from build123d import *

# Parameters (mm, degrees)
BOSS_EXTRUDE2_DEPTH = 48.5
BOSS_EXTRUDE3_DEPTH = 18
SKETCH3_R           = 1.6
CUT_EXTRUDE1_DEPTH  = 8
CUT_EXTRUDE3_DEPTH  = 3
SKETCH5_W           = 78.5
SKETCH5_H           = 16
BOSS_EXTRUDE4_DEPTH = 2
BOSS_EXTRUDE5_DEPTH = 7
BOSS_EXTRUDE6_DEPTH = 7
SKETCH10_R          = 2.1
CUT_EXTRUDE4_DEPTH  = 17
CUT_EXTRUDE5_DEPTH  = 3
CUT_EXTRUDE6_DEPTH  = 8


with BuildPart() as part:
    # Sketch1 → Boss-Extrude2 (new body)
    with BuildSketch(Plane.XY):
        with BuildLine():
            ThreePointArc((-2.027849528, -2.111075236), (-1.295616481, -3.878842189), (0.472150472, -4.611075236))
            Line((0.472150472, -4.611075236), (0.472150472, -7.611075236))
            Line((0.472150472, -7.611075236), (-17.527849528, -7.611075236))
            Line((-17.527849528, -7.611075236), (-17.527849528, 8.388924764))
            Line((-17.527849528, 8.388924764), (0.472150472, 8.388924764))
            Line((0.472150472, 8.388924764), (0.472150472, 5.388924764))
            ThreePointArc((0.472150472, 5.388924764), (-1.295616481, 4.656691717), (-2.027849528, 2.888924764))
            Line((-2.027849528, 2.888924764), (-2.027849528, -2.111075236))
        make_face()
    extrude(amount=BOSS_EXTRUDE2_DEPTH)

    # Sketch2 → Boss-Extrude3 (add)
    with BuildSketch(Plane.ZY.offset(17.527849528)):
        with BuildLine():
            Line((48.5, 8.388924764), (62.5, 8.388924764))
            Line((62.5, 8.388924764), (63.5, 8.388924764))
            Line((63.5, 8.388924764), (63.5, 7.388924764))
            Line((63.5, 7.388924764), (63.5, -6.611075236))
            Line((63.5, -6.611075236), (63.5, -7.611075236))
            Line((63.5, -7.611075236), (62.5, -7.611075236))
            Line((62.5, -7.611075236), (48.5, -7.611075236))
            Line((48.5, -7.611075236), (48.5, -4.811075236))
            Line((48.5, -4.811075236), (58.6, -4.811075236))
            ThreePointArc((58.6, -4.811075236), (58.670710678, -4.781785914), (58.7, -4.711075236))
            Line((58.7, -4.711075236), (58.7, 5.488924764))
            ThreePointArc((58.7, 5.488924764), (58.670710678, 5.559635442), (58.6, 5.588924764))
            Line((58.6, 5.588924764), (48.5, 5.588924764))
            Line((48.5, 5.588924764), (48.5, 8.388924764))
        make_face()
        with BuildLine():
            Line((0, -4.811075236), (0, -7.611075236))
            Line((0, -7.611075236), (-14, -7.611075236))
            Line((-14, -7.611075236), (-15, -7.611075236))
            Line((-15, -7.611075236), (-15, -6.611075236))
            Line((-15, -6.611075236), (-15, 7.388924764))
            Line((-15, 7.388924764), (-15, 8.388924764))
            Line((-15, 8.388924764), (-14, 8.388924764))
            Line((-14, 8.388924764), (0, 8.388924764))
            Line((0, 8.388924764), (0, 5.588924764))
            Line((0, 5.588924764), (-10.1, 5.588924764))
            ThreePointArc((-10.1, 5.588924764), (-10.170710678, 5.559635442), (-10.2, 5.488924764))
            Line((-10.2, 5.488924764), (-10.2, -4.711075236))
            ThreePointArc((-10.2, -4.711075236), (-10.170710678, -4.781785914), (-10.1, -4.811075236))
            Line((-10.1, -4.811075236), (0, -4.811075236))
        make_face()
    extrude(amount=-BOSS_EXTRUDE3_DEPTH)

    # Sketch3 → Cut-Extrude1 (cut)
    with BuildSketch(Plane.XY.offset(63.5)):
        with Locations((-9.527849528, 0.388924764)):
            Circle(SKETCH3_R)
    cut_extrude1 = extrude(amount=-CUT_EXTRUDE1_DEPTH, mode=Mode.SUBTRACT)

    # Mirror1: Cut-Extrude1 across plane
    add(cut_extrude1.mirror(Plane.XY.offset(24.25)), mode=Mode.SUBTRACT)

    # Sketch4 → Cut-Extrude3 (cut)
    with BuildSketch(Plane.XY.offset(63.5)):
        Polygon((-7.807950928, -2.618058576), (-6.063776267, 0.374908974), (-7.783674867, 3.381892314), (-11.247748128, 3.395908104), (-12.991922789, 0.402940554), (-11.272024189, -2.604042786), align=None)
    cut_extrude3 = extrude(amount=-CUT_EXTRUDE3_DEPTH, mode=Mode.SUBTRACT)

    # Mirror2: Cut-Extrude3 across plane
    add(cut_extrude3.mirror(Plane.XY.offset(24.25)), mode=Mode.SUBTRACT)

    # Sketch5 → Boss-Extrude4 (add)
    with BuildSketch(Plane.ZY.offset(17.527849528)):
        with Locations((24.25, 0.388924764)):
            Rectangle(SKETCH5_W, SKETCH5_H)
    extrude(amount=BOSS_EXTRUDE4_DEPTH)

    # Sketch6 → Boss-Extrude5 (add)
    with BuildSketch(Plane.XY.offset(63.5)):
        with BuildLine():
            Line((-19.527849528, -7.611075236), (-19.527849528, -8.257098609))
            ThreePointArc((-19.527849528, -8.257098609), (-29.816107458, -10.948302934), (-39.527849528, -15.28107317))
            Line((-39.527849528, -15.28107317), (-39.527849528, -18.149551009))
            ThreePointArc((-39.527849528, -18.149551009), (-8.277849528, -9.776138745), (22.972150472, -18.149551009))
            Line((22.972150472, -18.149551009), (22.972150472, -15.28107317))
            ThreePointArc((22.972150472, -15.28107317), (12.062731895, -10.540729559), (0.472150472, -7.867773606))
            Line((0.472150472, -7.867773606), (0.472150472, -7.611075236))
            Line((0.472150472, -7.611075236), (-19.527849528, -7.611075236))
        make_face()
    boss_extrude5 = extrude(amount=-BOSS_EXTRUDE5_DEPTH)

    # Mirror3: Boss-Extrude5 across plane
    add(boss_extrude5.mirror(Plane.XY.offset(24.25)))

    # Sketch7 → Boss-Extrude6 (add)
    with BuildSketch(Plane.XY.offset(63.5)):
        with BuildLine():
            Line((22.972150472, -18.149551009), (22.972150472, -15.28107317))
            ThreePointArc((22.972150472, -15.28107317), (28.129444831, -18.429050454), (32.972150472, -22.042310502))
            Line((32.972150472, -22.042310502), (32.972150472, -25.322038818))
            ThreePointArc((32.972150472, -25.322038818), (28.149113636, -21.489069971), (22.972150472, -18.149551009))
        make_face()
        with BuildLine():
            Line((-39.527849528, -15.28107317), (-39.527849528, -18.149551009))
            ThreePointArc((-39.527849528, -18.149551009), (-44.704812692, -21.489069971), (-49.527849528, -25.322038818))
            Line((-49.527849528, -25.322038818), (-49.527849528, -22.042310502))
            ThreePointArc((-49.527849528, -22.042310502), (-44.685143887, -18.429050454), (-39.527849528, -15.28107317))
        make_face()
    boss_extrude6 = extrude(amount=-BOSS_EXTRUDE6_DEPTH)

    # Mirror4: Boss-Extrude6 across plane
    add(boss_extrude6.mirror(Plane.XY.offset(24.25)))

    # Sketch10 → Cut-Extrude4 (cut, through all)
    with BuildSketch(Plane.XZ.offset(7.611075236)):
        with Locations((-9.527849528, 40.375)):
            Circle(SKETCH10_R)
        with Locations((-9.527849528, 8.125)):
            Circle(SKETCH10_R)
        with Locations((-9.527849528, 24.25)):
            Circle(SKETCH10_R)
    extrude(amount=-CUT_EXTRUDE4_DEPTH, mode=Mode.SUBTRACT)

    # Sketch11 → Cut-Extrude5 (cut)
    with BuildSketch(Plane(origin=(0, 8.388924764, 0), x_dir=(1, 0, 0), z_dir=(0, 1, 0))):
        Polygon((-7.751015125, -27.223694588), (-6.06413727, -24.198063563), (-7.840971673, -21.224368975), (-11.304683931, -21.276305412), (-12.991561786, -24.301936437), (-11.214727383, -27.275631025), align=None)
        Polygon((-7.751015125, -11.098694588), (-6.06413727, -8.073063563), (-7.840971673, -5.099368975), (-11.304683931, -5.151305412), (-12.991561786, -8.176936437), (-11.214727383, -11.150631025), align=None)
        Polygon((-7.751015125, -43.348694588), (-6.06413727, -40.323063563), (-7.840971673, -37.349368975), (-11.304683931, -37.401305412), (-12.991561786, -40.426936437), (-11.214727383, -43.400631025), align=None)
    extrude(amount=-CUT_EXTRUDE5_DEPTH, mode=Mode.SUBTRACT)

    # Sketch12 → Cut-Extrude6 (cut, through all)
    with BuildSketch(Plane.XY.offset(-8)):
        with BuildLine():
            Line((5.472150472, -8.747109948), (5.472150472, -11.307396754))
            ThreePointArc((5.472150472, -11.307396754), (20.100884553, -16.590436344), (32.972150472, -25.322038818))
            Line((32.972150472, -25.322038818), (32.972150472, -22.042310502))
            ThreePointArc((32.972150472, -22.042310502), (20.014209242, -13.756403523), (5.472150472, -8.747109948))
        make_face()
    extrude(amount=-CUT_EXTRUDE6_DEPTH, mode=Mode.SUBTRACT)


solid = part.part
Check sheet for the modelled part. Datum: model origin and axes. Units: mm. A direction names the side the tool comes from. Round coordinates to 2 decimals unless told otherwise and drop trailing zeros. Write each loop counter-clockwise with the first axis right and the second up, starting at its lowest first coordinate (ties: lowest second). Pieces come first, ordered by that corner, then holes. Notation, with made-up numbers: (-29.75, -16.75) -> (5.25, -16.75) arc R13 cw to (5.25, 8.25) -> close; hole circle Ø5 at (59, -17). An arc over 180 degrees is marked (long way). Answer as CSV lines item,"result". Start each with the question number.
1) Section check D-D on x = 14. Enter the section's corners in (y, z).
2) Section check B-B on x = -37. Enter the section's corners in (y, z).
3) Go/stop test with flat-tipped pins: P1, Ø19.5, axis at x = -13.5, y = -12, coming from the +Z side; P2, Ø5, axis at x = -9.53, y = 0.39, coming from the +Z side; P3, Ø5, axis at y = -0.5, z = 52, coming from the +X side; P4, Ø11, axis at y = -2, z = -3.5, coming from the +X side. Record where each tip stops, or that it passes through.
4) Section check C-C on y = -20. Enter the section's corners in (x, z), and give its area (3 significant figures).
5) Material ranges on line 1 (X direction, y = 4, z = 24.5); line 2 (X direction, y = 2, z = 0.5); line 3 (Z direction, x = 10, y = -10.5), recorded low to high. Write a range as from..to.
6) Section check A-A on z = 52. Enter the section's corners in (x, y).
7) Tool access check on faces 1 (the flat face through (-12.11, 1.92, 62.02)), 2 (the flat face through (-8, -9, 56.5)), 3 (the flat face through (-6.948, -1.143, -13.521)), 4 (the flat face through (-7, 5.389, 8)). Record the directions out of +Z, -Z, +X, -X, +Y, -Y that give a thin tool (end or side, any length) a straight path to the whole face; none if there is none.
8) Release check for a two-part mould opening along Z. For faces 5 (the flat face through (-2.028, 0, 24)), 6 (the flat face through (-8, 2, 60.5)), 7 (the flat face through (-14, -5, -15)) record: pulls with the +Z half, pulls with the -Z half, needs draft (parallel to the pull), parting line crosses it, or undercut.
Found:
1,outline,"(-13.88, 56.5) -> (-11.21, 56.5) -> (-11.21, 63.5) -> (-13.88, 63.5) -> close"
2,outline,"(-16.77, -15) -> (-13.97, -15) -> (-13.97, -8) -> (-16.77, -8) -> close; (-16.77, 56.5) -> (-13.97, 56.5) -> (-13.97, 63.5) -> (-16.77, 63.5) -> close"
3,P1,"stops at z = 63.5"
3,P2,"stops at z = 60.5"
3,P3,"stops at x = -17.53"
3,P4,"stops at x = 0.47"
4,outline,"(-46.91, -15) -> (-42.53, -15) -> (-42.53, -8) -> (-46.91, -8) -> close; (-46.91, 56.5) -> (-42.53, 56.5) -> (-42.53, 63.5) -> (-46.91, 63.5) -> close; (25.98, 56.5) -> (30.35, 56.5) -> (30.35, 63.5) -> (25.98, 63.5) -> close"
4,area,"91.8 mm^2"
5,line 1,"x = -19.53..-11.61, -7.44..-1.77"
5,line 2,"x = -19.53..-2.03"
5,line 3,"z = 56.5..63.5"
6,outline,"(-19.53, -7.61) -> (0.47, -7.61) -> (0.47, -4.81) -> (-17.53, -4.81) -> (-17.53, 5.59) -> (0.47, 5.59) -> (0.47, 8.39) -> (-19.53, 8.39) -> close"
7,face 1,"+Z"
7,face 2,"+X, -X, -Y"
7,face 3,"-Z"
7,face 4,"+Y"
8,face 5,"undercut"
8,face 6,"pulls with the +Z half"
8,face 7,"pulls with the -Z half"
